```python
from build123d import *

# Parameters (mm, degrees)
CYLINDER080_R          = 2
CYLINDER080_DEPTH      = 10
CYLINDER081_R          = 2
CYLINDER081_DEPTH      = 10
CYLINDER079_R          = 2
CYLINDER079_DEPTH      = 10
CYLINDER078_R          = 2
CYLINDER078_DEPTH      = 10
CYLINDER077_R          = 4
CYLINDER077_DEPTH      = 60
CYLINDER082_R          = 7.6
CYLINDER082_DEPTH      = 40
BOX027_W               = 25
BOX027_H               = 25
BOX027_DEPTH           = 5.2
CUT062_PLACEMENT_ANGLE = 90


with BuildPart() as cylinder080:
    # Cylinder080 → Cylinder080 (new body)
    with BuildSketch(Plane(origin=(21, 21, -2), x_dir=(1, 0, 0), z_dir=(0, 0, 1))):
        Circle(CYLINDER080_R)
    extrude(amount=CYLINDER080_DEPTH)


with BuildPart() as cylinder081:
    # Cylinder081 → Cylinder081 (new body)
    with BuildSketch(Plane(origin=(21, 4, -2), x_dir=(1, 0, 0), z_dir=(0, 0, 1))):
        Circle(CYLINDER081_R)
    extrude(amount=CYLINDER081_DEPTH)


with BuildPart() as cylinder079:
    # Cylinder079 → Cylinder079 (new body)
    with BuildSketch(Plane(origin=(4, 21, -2), x_dir=(1, 0, 0), z_dir=(0, 0, 1))):
        Circle(CYLINDER079_R)
    extrude(amount=CYLINDER079_DEPTH)


with BuildPart() as cylinder078:
    # Cylinder078 → Cylinder078 (new body)
    with BuildSketch(Plane(origin=(4, 4, -2), x_dir=(1, 0, 0), z_dir=(0, 0, 1))):
        Circle(CYLINDER078_R)
    extrude(amount=CYLINDER078_DEPTH)


with BuildPart() as cylinder077:
    # Cylinder077 → Cylinder077 (new body)
    with BuildSketch(Plane(origin=(12.5, 12.5, -7), x_dir=(1, 0, 0), z_dir=(0, 0, 1))):
        Circle(CYLINDER077_R)
    extrude(amount=CYLINDER077_DEPTH)


with BuildPart() as cylinder082:
    # Cylinder082 → Cylinder082 (new body)
    with BuildSketch(Plane(origin=(12.5, 12.5, 5), x_dir=(1, 0, 0), z_dir=(0, 0, 1))):
        Circle(CYLINDER082_R)
    extrude(amount=CYLINDER082_DEPTH)


with BuildPart() as cut062:
    # Box027 → Box027 (new body)
    with BuildSketch(Plane.XY):
        with Locations((12.5, 12.5)):
            Rectangle(BOX027_W, BOX027_H)
    extrude(amount=BOX027_DEPTH)

    # Fusion034: union Cylinder082
    add(cylinder082.part)

    # Cut060: cut Cylinder077
    add(cylinder077.part, mode=Mode.SUBTRACT)

    # Cut061: cut Cylinder078
    add(cylinder078.part, mode=Mode.SUBTRACT)

    # Cut058: cut Cylinder079
    add(cylinder079.part, mode=Mode.SUBTRACT)

    # Cut059: cut Cylinder081
    add(cylinder081.part, mode=Mode.SUBTRACT)

    # Cut062: cut Cylinder080
    add(cylinder080.part, mode=Mode.SUBTRACT)


with BuildPart() as cut062_1:
    # Cut062 placement: moved
    add(cut062.part.moved(Location((-12.5, 0, 12.5))).rotate(Axis((-12.5, 0, 12.5), (-1, 0, 0)), CUT062_PLACEMENT_ANGLE))


solid = cut062_1.part
```
Here's how the part is built. I have some questions about the finished solid (model axes, mm). A direction names the side the tool comes from. Round coordinates to 2 decimals unless told otherwise and drop trailing zeros. Order: outer loops, then holes, each group sorted by start corner. A loop starts at its lowest first (then second) coordinate and runs counter-clockwise, first axis right, second up. Notation, with made-up numbers: M 1,59.5 L 48,59.5 A38 ccw 48,98.5 Z; hole C -5.75,58 d5. An arc over 180 degrees is marked long. Answer as CSV lines item,"result".
Item 1: Please list where these lines run through material, in increasing order: L1, parallel to Z at x = 8.5, y = 3.3; L2, parallel to Z at x = 0, y = 33; L3, parallel to Y at x = -2, z = 11.25. Write a range as [from, to].
From the geometry:
L1,"[-12.5, -10.5], [-6.5, 6.5], [10.5, 12.5]"
L2,"[-7.6, -4], [4, 7.6]"
L3,"[0, 5.2]"
Item 2: Imagine slicing it at C-C on x = 0. List the corners of the cut face in (y, z) for me.
From the geometry:
outline,"M 0,-12.5 L 5.2,-12.5 L 5.2,-7.6 L 45,-7.6 L 45,-4 L 0,-4 Z; M 0,4 L 45,4 L 45,7.6 L 5.2,7.6 L 5.2,12.5 L 0,12.5 Z"
Item 3: For pin 1 (1 mm diameter, centred on x = 5.5, y = 37.5, fed in from +Z); pin 2 (1.5 mm diameter, centred on y = 8, z = 9, fed in from -X); pin 3 (8 mm diameter, centred on y = 15, z = 1.5, fed in from -X); pin 4 (8 mm diameter, centred on y = 22, z = -7.5, fed in from +X), each with a flat end and sliding along its axis, tell me the tip position at first contact or that it passes through.
From the geometry:
pin 1,"z = 5.72"
pin 2,"through"
pin 3,"x = -7.6"
pin 4,"x = 6.75"
Item 4: Imagine slicing it at D-D on y = 3. List the corners of the cut face in (x, z) for me, and give its area (3 significant figures).
From the geometry:
outline,"M -12.5,-12.5 L 12.5,-12.5 L 12.5,12.5 L -12.5,12.5 Z; hole C -8.5,-8.5 d4; hole C -8.5,8.5 d4; hole C 0,0 d8; hole C 8.5,-8.5 d4; hole C 8.5,8.5 d4"
area,"524 mm2"
Item 5: Which directions (+Z, -Z, +X, -X, +Y, -Y) give clear straight access to the entire face, cutting with the end or side of a thin tool? Please do faces 5 (the cylindrical face through (7.026, 2.564, 7.148)), 6 (the cylindrical face through (4.1, 24.8, -6.4)).
From the geometry:
face 5,"+Y, -Y"
face 6,"+Y"
Item 6: Imagine slicing it at A-A on x = 8.5. List the corners of the cut face in (y, z) for me, and give its area (3 significant figures).
From the geometry:
outline,"M 0,-12.5 L 5.2,-12.5 L 5.2,-10.5 L 0,-10.5 Z; M 0,-6.5 L 5.2,-6.5 L 5.2,6.5 L 0,6.5 Z; M 0,10.5 L 5.2,10.5 L 5.2,12.5 L 0,12.5 Z"
area,"88.4 mm2"
Item 7: We'd pull the mould along X, two halves only. Please class faces 1 (the flat face through (-3, 0, -3)), 2 (the flat face through (-12.5, 3, 0)), 3 (the flat face through (12.5, 3, 0)), 4 (the cylindrical face through (-9.974, 2.564, 7.148)): +X half, -X half, draft (parallel to the pull), parting line (faces both ways), or undercut.
From the geometry:
face 1,"draft"
face 2,"-X half"
face 3,"+X half"
face 4,"undercut"
Item 8: Imagine slicing it at B-B on z = 8.5. List the corners of the cut face in (x, y) for me.
From the geometry:
outline,"M -12.5,0 L -10.5,0 L -10.5,5.2 L -12.5,5.2 Z; M -6.5,0 L 6.5,0 L 6.5,5.2 L -6.5,5.2 Z; M 10.5,0 L 12.5,0 L 12.5,5.2 L 10.5,5.2 Z"
